Part model, mm, in its own coordinate system. A direction names the side the tool comes from. Coordinates: 2 decimals unless noted, no trailing zeros. Write each loop counter-clockwise with the first axis right and the second up, starting at its lowest first coordinate (ties: lowest second). Pieces come first, ordered by that corner, then holes. Notation, with made-up numbers: M 10,-28.75 L 59,-28.75 A36 cw 59,6.25 Z; hole C 58,88.5 d6. An arc over 180 degrees is marked long. Use a Markdown table: item, result. Add a question column.
Q1. Tool access for faces 1 (the flat face through (99, -400, 10)), 2 (the flat face through (170, -260, 10)): list every direction of +Z, -Z, +X, -X, +Y, -Y with a clear straight run to the whole face (end or side of a thin tool).
Q2. Pin check, flat tips, straight feed: pin 1 Ø2.5 at (x, y) = (143, -200) entering from +Z; pin 2 Ø2 at (y, z) = (-226, 4) entering from +X; pin 3 Ø1.8 at (y, z) = (-202, 10.5) entering from +X. Stop position of each tip, or through.
Q3. Wall check: L1, parallel to Y at x = 165, z = 12.75; L2, parallel to X at y = -141, z = 5.25. Give the ranges that are in metal, low to high. Write a range as from..to.
Q4. Slice it at C-C on y = -234.5. Write the cut outline in (x, z), then the cut area to 3 significant figures.
Q5. Slice it at B-B on z = 16.75. Write the cut outline in (x, y).
Q6. Slice it at A-A on x = 165.5. Write the cut outline in (y, z).
from build123d import *

# Parameters (mm, degrees)
F0_W     = 200
F0_H     = 20
F1_DEPTH = 400
F3_DEPTH = 25
F4_W     = 10
F4_H     = 6
F5_DEPTH = 5


with BuildPart() as f1:
    # F0 (on Front) → F1 (new body)
    with BuildSketch(Plane.XZ):
        with Locations((100, 10)):
            Rectangle(F0_W, F0_H)
    extrude(amount=F1_DEPTH)

    # F2 (on face) → F3 (cut)
    with BuildSketch(Plane.XY.offset(20)):
        Polygon((200, -260), (200, -200), (200, -140), (140, -140), (140, -260), align=None)
    extrude(amount=-F3_DEPTH, mode=Mode.SUBTRACT)

    # F4 (on face) → F5 (join)
    with BuildSketch(Plane.YZ.offset(140)):
        with Locations((-200, 10)):
            Rectangle(F4_W, F4_H)
    extrude(amount=F5_DEPTH)


solid = f1.part
Recorded:
| question | item | result |
|---|---|---|
| 1 | face 1 | +Z, -Z, +X, -X, -Y |
| 1 | face 2 | +Z, -Z, +X |
| 2 | pin 1 | z = 13 |
| 2 | pin 2 | x = 140 |
| 2 | pin 3 | x = 145 |
| 3 | L1 | -400..-260, -140..0 |
| 3 | L2 | 0..140 |
| 4 | outline | M 0,0 L 140,0 L 140,20 L 0,20 Z |
| 4 | area | 2,800 mm² |
| 5 | outline | M 0,-400 L 200,-400 L 200,-260 L 140,-260 L 140,-140 L 200,-140 L 200,0 L 0,0 Z |
| 6 | outline | M -400,0 L -260,0 L -260,20 L -400,20 Z; M -140,0 L 0,0 L 0,20 L -140,20 Z |
